Model file for the job. Use its own axes, mm. Round coordinates to 2 decimals unless told otherwise and drop trailing zeros. Write each loop counter-clockwise with the first axis right and the second up, starting at its lowest first coordinate (ties: lowest second). Pieces come first, ordered by that corner, then holes.
```python
from build123d import *

# Parameters (mm, degrees)
SKETCH1_R           = 2
BOSS_EXTRUDE1_DEPTH = 1.5


with BuildPart() as part:
    # Sketch1 → Boss-Extrude1 (new, symmetric)
    with BuildSketch(Plane(origin=(0, 0, 0), x_dir=(1, 0, 0), z_dir=(0, 1, 0))):
        with BuildLine():
            Line((-6.312384572, -84.941682553), (-6.312384976, -84.943885306))
            ThreePointArc((-6.312384976, -84.943885306), (-0.312384976, -90.943885306), (5.687615024, -84.943885306))
            Line((5.687615024, -84.943885306), (5.687615024, 85.184041034))
            ThreePointArc((5.687615024, 85.184041034), (-0.617919518, 91.176256705), (-6.281267857, 84.573764744))
            Line((-6.281267857, 84.573764744), (-6.312384572, -84.941682553))
        make_face()
        with Locations(Location((-0.312384976, -84.943885306, 0), (0, 0, 270))):
            Circle(SKETCH1_R, mode=Mode.SUBTRACT)
        with Locations(Location((-0.312384976, 85.184041034, 0), (0, 0, 270))):
            Circle(SKETCH1_R, mode=Mode.SUBTRACT)
    extrude(amount=BOSS_EXTRUDE1_DEPTH, both=True)


solid = part.part
```
1) Pull direction Z, two halves, no side cores. Call faces 1 (the face through (0.288, -0.021, -83.276)), 2 (the face through (-0.444, 0.021, 90.942)), 3 (the face through (5.688, 0, 1)): released by +Z, released by -Z, zero draft, split by the parting line, or undercut.
2) Wall check: probe 1 along Z at (x, y) = (0, 0.45); probe 2 along Z at (x, y) = (1, 0.85); probe 3 along X at (y, z) = (0, -46). Give the ranges that are in metal, low to high.
3) Cut at A-A on y = 0.25. Give the number of separate pieces and of enclosed holes in the cut face, and give its area (3 significant figures).
4) Cut at B-B on x = 3.5. List the corners of the cut face in (y, z).
5) Flat gauge pins, fed straight in: pin 1 Ø1.5 at (x, y) = (2, 0.5) entering from -Z; pin 2 Ø3 at (x, z) = (-0.31, 84.94) entering from -Y. Where does each tip first touch, or does it go through?
Result sheet:
1. face 1: undercut
1. face 2: released by +Z
1. face 3: zero draft
2. probe 1: z = -91.18 to -87.16, -83.21 to 82.97, 86.92 to 90.94
2. probe 2: z = -91.04 to -86.69, -83.67 to 83.43, 86.45 to 90.8
2. probe 3: x = -6.29 to 5.69
3. separate pieces: 1
3. enclosed holes: 2
3. area: 2,130 mm2
4. outline: (-1.5, -89.82) - (1.5, -89.82) - (1.5, 89.58) - (-1.5, 89.58) - close
5. pin 1: stops at z = -90.98
5. pin 2: passes through
